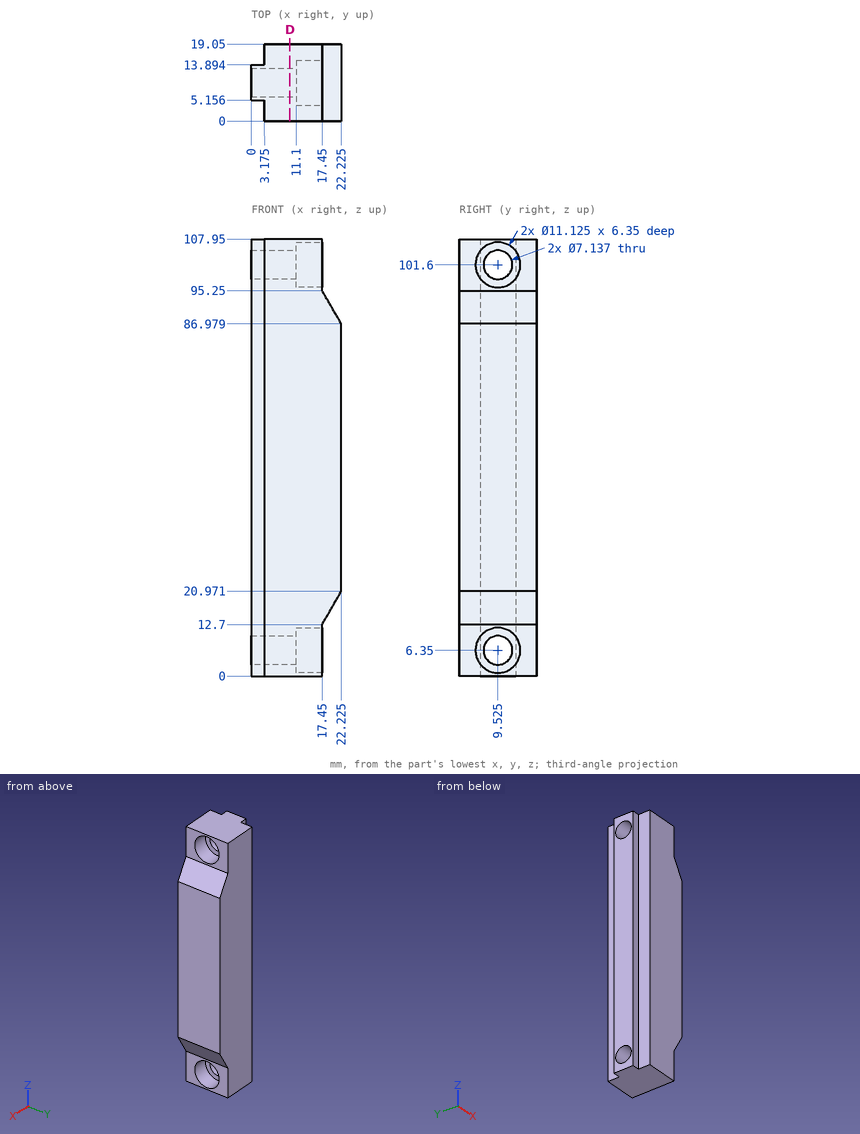
Part print with two shaded views. Sizes in mm from the minimum x, y, z corner. Coordinates: 2 decimals unless noted, no trailing zeros. Answer in a Markdown table with one row per item.
1. Flat gauge pins, fed straight in: P1, Ø1.6, axis at x = 1.5, z = 33.5, coming from the -Y side; P2, Ø10, axis at y = 9.525, z = 101.6, coming from the +X side; P3, Ø4, axis at y = 2.5, z = 45.5, coming from the -X side (3 decimals). Where does each tip first touch, or does it go through?
Answer:
| item | result |
|---|---|
| P1 | y = 5.16 |
| P2 | x = 11.1 |
| P3 | x = 3.175 |
2. Drill centre lines: L1, parallel to Y at x = 13.5, z = 101.6; L2, parallel to Y at x = 5.75, z = 101.6; L3, parallel to Z at x = 10.5, y = 11.5. Where is each one in solid material? Low to high. Write a range as from..to.
Answer:
| item | result |
|---|---|
| L1 | 0..3.96, 15.09..19.05 |
| L2 | 0..5.96, 13.09..19.05 |
| L3 | 0..3.38, 9.32..98.63, 104.57..107.95 |
3. Slice it at D-D, the plane x = 9.5. Give the number of separate pieces and of enclosed holes in the cut face, then the cut area to 3 significant figures.
Answer:
| item | result |
|---|---|
| separate pieces | 1 |
| enclosed holes | 2 |
| area | 1,980 mm² |
